Check sheet for the modelled part. Datum: model origin and axes. Units: mm. Face numbers are marked on the shaded views. A direction names the side the tool comes from. Give positions to 0.01 mm unless a question says otherwise; leave off trailing zeros. Order: outer loops, then holes, each group sorted by start corner. A loop starts at its lowest first (then second) coordinate and runs counter-clockwise, first axis right, second up. Notation, with made-up numbers: M 4.25,12 L 31.25,12 A14 cw 31.25,37 Z; hole C -31,61 d8. An arc over 180 degrees is marked long. Answer in a Markdown table with one row per item. Add a question column.
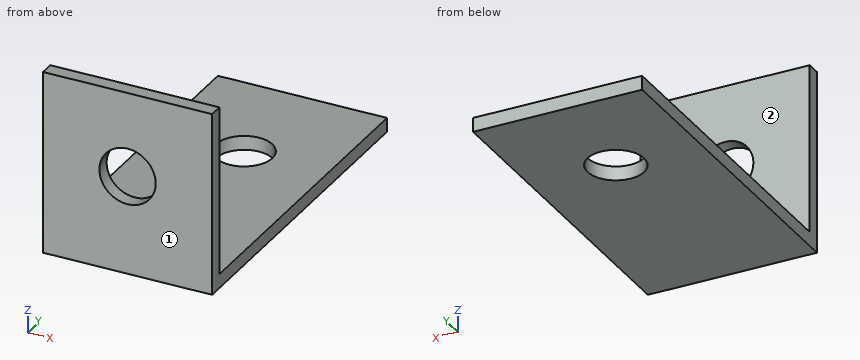
from build123d import *

# Parameters (mm, degrees)
SKETCH1_W           = 19.05
SKETCH1_H           = 38.1
SKETCH1_R           = 3.175
BOSS_EXTRUDE1_DEPTH = 0.79375
SKETCH2_W           = 19.05
SKETCH2_H           = 19.05
SKETCH2_R           = 3.175
BOSS_EXTRUDE2_DEPTH = 1.5875


with BuildPart() as part:
    # Sketch1 → Boss-Extrude1 (new body, symmetric)
    with BuildSketch(Plane.XY):
        Rectangle(SKETCH1_W, SKETCH1_H)
        with Locations((0, 6.35)):
            Circle(SKETCH1_R, mode=Mode.SUBTRACT)
    extrude(amount=BOSS_EXTRUDE1_DEPTH, both=True)

    # Sketch2 → Boss-Extrude2 (add)
    with BuildSketch(Plane.XZ.offset(19.05)):
        with Locations((0, 10.31875)):
            Rectangle(SKETCH2_W, SKETCH2_H)
        with Locations((0, 10.31875)):
            Circle(SKETCH2_R, mode=Mode.SUBTRACT)
    extrude(amount=-BOSS_EXTRUDE2_DEPTH)


solid = part.part
Q1. Cross-section at D-D (x = 2). Record the boundary of the cut face in (y, z).
Q2. Thickness scan on probe 1 along Y at (x, z) = (0, 0.3) (3 decimals); probe 2 along Z at (x, y) = (0, -18.45); probe 3 along Y at (x, z) = (0.75, 18). Record the ranges inside material, lowest first.
Q3. Go/stop test with flat-tipped pins: pin 1 (1 mm diameter, centred on x = 0, z = 9, fed in from +Y); pin 2 (6 mm diameter, centred on x = 0, y = -7.5, fed in from +Z). Record where each tip stops, or that it passes through.
Q4. Tool access check on the marked faces 1 and 2. Record the directions out of +Z, -Z, +X, -X, +Y, -Y that give a thin tool (end or side, any length) a straight path to the whole face; none if there is none.
Q5. Cross-section at A-A (y = 6.35). Record the boundary of the cut face in (x, z) (3 decimals), and give its area (3 significant figures).
Q6. Cross-section at B-B (x = -0.75). Record the boundary of the cut face in (y, z), and give its area (3 significant figures).
Values follow:
| question | item | result |
|---|---|---|
| 1 | outline | M -19.05,-0.79 L 3.88,-0.79 L 3.88,0.79 L -17.46,0.79 L -17.46,7.85 L -19.05,7.85 Z; M -19.05,12.78 L -17.46,12.78 L -17.46,19.84 L -19.05,19.84 Z; M 8.82,-0.79 L 19.05,-0.79 L 19.05,0.79 L 8.82,0.79 Z |
| 2 | probe 1 | -19.05 to 3.175, 9.525 to 19.05 |
| 2 | probe 2 | -0.79 to 7.14, 13.49 to 19.84 |
| 2 | probe 3 | -19.05 to -17.46 |
| 3 | pin 1 | through |
| 3 | pin 2 | z = 0.79 |
| 4 | face 1 | +Z, -Z, +X, -X, -Y |
| 4 | face 2 | +Z, +X, -X, +Y |
| 5 | outline | M -9.525,-0.794 L -3.175,-0.794 L -3.175,0.794 L -9.525,0.794 Z; M 3.175,-0.794 L 9.525,-0.794 L 9.525,0.794 L 3.175,0.794 Z |
| 5 | area | 20.2 mm² |
| 6 | outline | M -19.05,-0.79 L 3.26,-0.79 L 3.26,0.79 L -17.46,0.79 L -17.46,7.23 L -19.05,7.23 Z; M -19.05,13.4 L -17.46,13.4 L -17.46,19.84 L -19.05,19.84 Z; M 9.44,-0.79 L 19.05,-0.79 L 19.05,0.79 L 9.44,0.79 Z |
| 6 | area | 71.1 mm² |
